Can you work these out from the model? Positions are in its coordinate system, mm. Face numbers are marked on the shaded views. A direction names the side the tool comes from. Round coordinates to 2 decimals unless told otherwise and drop trailing zeros. Loops run counter-clockwise (first coordinate to the right, second up) from the corner with the lowest first, then second, coordinate; pieces in that order, holes last. Notation, with made-up numbers: M 28.5,-12.75 L 58.5,-12.75 A9 cw 58.5,0.25 Z; hole C -25,79 d1. An arc over 180 degrees is marked long. Answer as CSV lines item,"result".
from build123d import *

# Parameters (mm, degrees)
SKETCH1_W           = 200
SKETCH1_H           = 100
BOSS_EXTRUDE1_DEPTH = 10
SKETCH2_W           = 40
SKETCH2_H           = 10
SKETCH2_W_2         = 10
SKETCH2_H_2         = 40
BOSS_EXTRUDE2_DEPTH = 40
SKETCH4_R           = 5
CUT_EXTRUDE2_DEPTH  = 31
SKETCH7_W           = 200
SKETCH7_H           = 10
BOSS_EXTRUDE3_DEPTH = 65
SKETCH9_R           = 5
CUT_EXTRUDE4_DEPTH  = 130


with BuildPart() as part:
    # Sketch1 → Boss-Extrude1 (new body)
    with BuildSketch(Plane.XY):
        Rectangle(SKETCH1_W, SKETCH1_H)
    extrude(amount=BOSS_EXTRUDE1_DEPTH)

    # Sketch2 → Boss-Extrude2 (add)
    with BuildSketch(Plane(origin=(0, 0, 0), x_dir=(-1, 0, 0), z_dir=(0, 0, -1))):
        with Locations((14, 0)):
            Rectangle(SKETCH2_W, SKETCH2_H)
        with Locations((95, 0)):
            Rectangle(SKETCH2_W_2, SKETCH2_H_2)
    extrude(amount=BOSS_EXTRUDE2_DEPTH)

    # Sketch4 → Cut-Extrude2 (cut)
    with BuildSketch(Plane.ZY.offset(100)):
        with Locations((-20, 0)):
            Circle(SKETCH4_R)
    extrude(amount=-CUT_EXTRUDE2_DEPTH, mode=Mode.SUBTRACT)

    # Sketch7 → Boss-Extrude3 (add, symmetric)
    with BuildSketch(Plane(origin=(0, 0, 0), x_dir=(1, 0, 0), z_dir=(0, 1, 0))):
        with Locations((0, -5)):
            Rectangle(SKETCH7_W, SKETCH7_H)
    extrude(amount=BOSS_EXTRUDE3_DEPTH, both=True)

    # Sketch9 → Cut-Extrude4 (cut)
    with BuildSketch(Plane(origin=(0, 5, 0), x_dir=(1, 0, 0), z_dir=(0, 1, 0))):
        with Locations((-14, 20)):
            Circle(SKETCH9_R)
    extrude(amount=-CUT_EXTRUDE4_DEPTH, mode=Mode.SUBTRACT)


solid = part.part
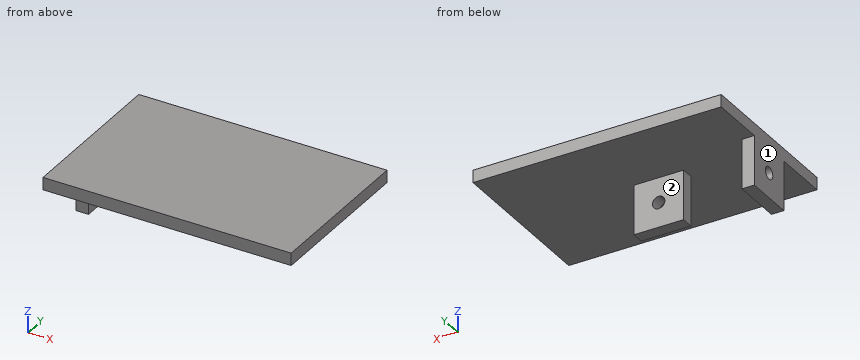
Item 1: If we section it at C-C on z = -29.5: Write out the boundary of the cut face in (x, y), then the cut area to 3 significant figures.
Output:
outline,"M -100,-20 L -90,-20 L -90,20 L -100,20 Z; M -34,-5 L 6,-5 L 6,5 L -34,5 Z"
area,"800 mm2"
Item 2: Will these pins go through, and if not, where does the flat tip stop? pin 1 (16 mm diameter, centred on x = -14, z = -20, fed in from +Y); pin 2 (3 mm diameter, centred on y = 1, z = -20, fed in from -X); pin 3 (8 mm diameter, centred on x = -95, z = -21.5, fed in from -Y).
Output:
pin 1,"stops at y = 5"
pin 2,"stops at x = -34"
pin 3,"stops at y = -20"
Item 3: If we section it at D-D on z = -20: Write out the boundary of the cut face in (x, y), then the cut area to 3 significant figures.
Output:
outline,"M -100,-20 L -90,-20 L -90,-5 L -100,-5 Z; M -100,5 L -90,5 L -90,20 L -100,20 Z; M -34,-5 L -19,-5 L -19,5 L -34,5 Z; M -9,-5 L 6,-5 L 6,5 L -9,5 Z"
area,"600 mm2"
Item 4: On a 3-axis mill with a long thin cutter (end or side, diameter ignored), from which of +Z, -Z, +X, -X, +Y, -Y can I reach the whole of each face in a straight line? I mean the marked faces 1 and 2. Say none if no direction works.
Output:
face 1,"+Z, -Z, -X, +Y, -Y"
face 2,"-Z, +X, +Y"
Item 5: If we section it at A-A on y = 0: Write out the boundary of the cut face in (x, z), then the cut area to 3 significant figures.
Output:
outline,"M -100,-40 L -90,-40 L -90,-25 L -100,-25 Z; M -100,-15 L -90,-15 L -90,0 L -34,0 L -34,-40 L 6,-40 L 6,0 L 100,0 L 100,10 L -100,10 Z; hole C -14,-20 d10"
area,"3,820 mm2"
Item 6: If we section it at B-B on x = -14: Write out the boundary of the cut face in (y, z), then the cut area to 3 significant figures.
Output:
outline,"M -65,0 L -5,0 L -5,-15 L 5,-15 L 5,0 L 65,0 L 65,10 L -65,10 Z; M -5,-40 L 5,-40 L 5,-25 L -5,-25 Z"
area,"1,600 mm2"
Item 7: If I drill on line 1 along X through (y, z) = (-2.5, -20); line 2 along Z through (x, y) = (-14, 2); line 3 along Y through (x, z) = (-94, -20), over which ranges is the centre line in solid material (lowest first)? Write a range as from..to.
Output:
line 1,"x = -34..-19, -9..6"
line 2,"z = -40..-25, -15..10"
line 3,"y = -20..-5, 5..20"
